from build123d import *

# Parameters (mm, degrees)
F0_R            = 14.1331511128
F0_R_2          = 1.8288
F1_DEPTH        = 6.35
F2_W            = 9.1077039159
F2_H            = 9.1077039159
F3_DEPTH        = 3.175
F4_R            = 6.4401192
F5_DEPTH        = 1.5875
F7_DEPTH        = 6.35
F7_COPIES_COUNT = 19


# Not quite as in the source:
# - a pattern or mirror of a feature is missing from the dataset's text; its kind, count and spacing are read off the source's solid


with BuildPart() as f1:
    # F0 (on Top) → F1 (new body)
    with BuildSketch(Plane.XY):
        Circle(F0_R)
        Circle(F0_R_2, mode=Mode.SUBTRACT)
    extrude(amount=F1_DEPTH)

    # F2 (on face) → F3 (cut)
    with BuildSketch(Plane(origin=(0, 0, 0), x_dir=(1, 0, 0), z_dir=(0, 0, -1))):
        Rectangle(F2_W, F2_H)
    extrude(amount=-F3_DEPTH, mode=Mode.SUBTRACT)

    # F4 (on face) → F5 (cut)
    with BuildSketch(Plane(origin=(0, 0, 0), x_dir=(1, 0, 0), z_dir=(0, 0, -1))):
        Circle(F4_R)
    extrude(amount=-F5_DEPTH, mode=Mode.SUBTRACT)

    # F6 (on face) → F7 (cut, through all)
    with BuildSketch(Plane.XY.offset(6.35)):
        with BuildLine():
            Line((0.4054121916, 11.2582715851), (1.6826301613, 14.0326304063))
            ThreePointArc((1.6826301613, 14.0326304063), (0, 14.1331511128), (-1.6826301613, 14.0326304063))
            Line((-1.6826301613, 14.0326304063), (-0.4054121916, 11.2582715851))
            ThreePointArc((-0.4054121916, 11.2582715851), (0, 10.9985991732), (0.4054121916, 11.2582715851))
        make_face()
    f7 = extrude(amount=-F7_DEPTH, mode=Mode.SUBTRACT)

    # F7_copies: F7 ×19 about axis
    f7_copies_axis = Axis((0, 0, 0), (0, 0, 1))
    for i in range(1, F7_COPIES_COUNT):
        add(f7.rotate(f7_copies_axis, i * 360 / F7_COPIES_COUNT), mode=Mode.SUBTRACT)


solid = f1.part
Here's how the part is built. I have some questions about the finished solid (model axes, mm). A direction names the side the tool comes from. Coordinates: 2 decimals unless noted, no trailing zeros. Loops run counter-clockwise (first coordinate to the right, second up) from the corner with the lowest first, then second, coordinate; pieces in that order, holes last.
1. If we mould it in two halves opening along X, with no side actions, what happens to faces 1 (the flat face through (-11.179, 6.046, 3.219)), 2 (the flat face through (-4.554, 0, 2)), 3 (the cylindrical face through (14.086, 1.158, 3.131)), 4 (the cylindrical face through (-4.598, -13.364, 3.131))? For each: pulls with the +X half, pulls with the -X half, needs draft (parallel to the pull), parting line crosses it, or undercut.
2. Imagine slicing it at C-C, the plane y = 9.5. Please give me the cut outline in (x, z), and give its area (3 significant figures).
3. For faces 5 (the flat face through (-6.94, 10.6, 3.22)), 6 (the flat face through (3.123, -12.319, 3.219)), 7 (the flat face through (-11.175, -6.052, 3.219)), 8 (the flat face through (-5.11, 11.64, 3.22)), which set-ups out of +Z, -Z, +X, -X, +Y, -Y let a thin tool reach every point of the face, with its end or its side?
4. For P1, Ø2.5, axis at x = 2, y = 1, coming from the -Z side (3 decimals); P2, Ø1.5, axis at x = 0, y = -6, coming from the -Z side; P3, Ø2, axis at x = 0.5, y = 5, coming from the -Z side; P4, Ø1, axis at x = 1, z = 3.5, coming from the -Y side, each with a flat end and sliding along its axis, tell me the tip position at first contact or that it passes through.
5. I need wall thicknesses on L1, parallel to X at y = 10.75, z = 5; L2, parallel to X at y = 9, z = 4.25; L3, parallel to Z at x = -2, y = 1.5 (3 decimals). Which ranges of each line are inside material? Lowest first, please.
Taken from the geometry:
1. face 1: undercut
1. face 2: undercut
1. face 3: pulls with the +X half
1. face 4: pulls with the -X half
2. outline: (-10.46, 0) - (-8.9, 0) - (-8.9, 6.35) - (-10.46, 6.35) - close; (-6.68, 0) - (6.68, 0) - (6.68, 6.35) - (-6.68, 6.35) - close; (8.9, 0) - (10.46, 0) - (10.46, 6.35) - (8.9, 6.35) - close
2. area: 105 mm2
3. face 5: +Z, -Z
3. face 6: +Z, -Z, -Y
3. face 7: +Z, -Z, -X
3. face 8: +Z, -Z, +Y
4. P1: stops at z = 3.175
4. P2: stops at z = 0
4. P3: stops at z = 1.59
4. P4: stops at y = -14.12
5. L1: x = -6.97 to -4.26, -3.28 to 3.28, 4.26 to 6.97
5. L2: x = -10.77 to -7.94, -6.58 to 6.58, 7.94 to 10.77
5. L3: z = 3.175 to 6.35
